from build123d import *

# Parameters (mm, degrees)
SKETCH1_W                = 40.386
SKETCH1_H                = 19.812
BOSS_EXTRUDE1_DEPTH      = 40.64
SKETCH2_W                = 19.812
SKETCH2_H                = 4
BOSS_EXTRUDE2_DEPTH      = 7
BOSS_EXTRUDE2_DEPTH_BACK = 47
SKETCH3_R                = 8.5
BOSS_EXTRUDE3_DEPTH      = 2
FILLET1_R                = 1
SKETCH4_R                = 2.117245373
BOSS_EXTRUDE4_DEPTH      = 5.2


with BuildPart() as part:
    # Sketch1 → Boss-Extrude1 (new body)
    with BuildSketch(Plane(origin=(0, 0, 0), x_dir=(1, 0, 0), z_dir=(0, 1, 0))):
        Rectangle(SKETCH1_W, SKETCH1_H)
    extrude(amount=BOSS_EXTRUDE1_DEPTH)

    # Sketch2 → Boss-Extrude2 (add, two sides)
    with BuildSketch(Plane(origin=(20.193, 0, 0), x_dir=(0, 0, -1), z_dir=(1, 0, 0))) as boss_extrude2_sk:
        with Locations((0, 25.94)):
            Rectangle(SKETCH2_W, SKETCH2_H)
    extrude(amount=BOSS_EXTRUDE2_DEPTH)
    extrude(boss_extrude2_sk.sketch, amount=-BOSS_EXTRUDE2_DEPTH_BACK)

    # Sketch3 → Boss-Extrude3 (add)
    with BuildSketch(Plane(origin=(0, 40.64, 0), x_dir=(1, 0, 0), z_dir=(0, 1, 0))):
        with Locations((10.018571985, 0)):
            Circle(SKETCH3_R)
    extrude(amount=BOSS_EXTRUDE3_DEPTH)

    # Fillet1
    fillet1_edges = [part.edges().sort_by_distance(p)[0] for p in [
        (1.518571985, 42.64, 0),
    ]]
    fillet(fillet1_edges, radius=FILLET1_R)

    # Sketch4 → Boss-Extrude4 (add)
    with BuildSketch(Plane(origin=(0, 42.64, 0), x_dir=(1, 0, 0), z_dir=(0, 1, 0))):
        with Locations((10.018571985, 0)):
            Circle(SKETCH4_R)
    extrude(amount=BOSS_EXTRUDE4_DEPTH)


solid = part.part
Can you work these out from the model? Positions are in its coordinate system, mm. A direction names the side the tool comes from. Coordinates: 2 decimals unless noted, no trailing zeros. Loops run counter-clockwise (first coordinate to the right, second up) from the corner with the lowest first, then second, coordinate; pieces in that order, holes last. Notation, with made-up numbers: M 82,0 L 140,0 A14 ccw 140,12 Z; hole C 10,-6 d8. An arc over 180 degrees is marked long. Answer as CSV lines item,"result". Start each with the question number.
1. Suppose I cut it at B-B, the plane x = 22.5. List the corners of the cut face in (y, z) for me.
2. For faces 1 (the face through (-23, 27.94, 0)), 2 (the face through (20.193, 34, 0)), 3 (the face through (-23, 23.94, 0)), 4 (the face through (12, 42.64, 2)), which set-ups out of +Z, -Z, +X, -X, +Y, -Y let a thin tool reach every point of the face, with its end or its side?
3. Suppose I cut it at C-C, the plane y = 38. List the corners of the cut face in (x, z) for me.
4. For pin 1 Ø7.5 at (x, z) = (24, -1) entering from -Y; pin 2 Ø3.5 at (x, z) = (-23.5, 0.5) entering from +Y; pin 3 Ø6 at (y, z) = (7, -5) entering from +X, each with a flat end and sliding along its axis, tell me the tip position at first contact or that it passes through.
5. If I drill on probe 1 along Y at (x, z) = (-8, 0); probe 2 along X at (y, z) = (12.5, 5); probe 3 along Y at (x, z) = (24, 4.5), over which ranges is the centre line in solid material (lowest first)? Write a range as [from, to].
6. Suppose I cut it at A-A, the plane z = 0. List the corners of the cut face in (x, y) for me, plus the area to 3 significant figures.
Output:
1,outline,"M 23.94,-9.91 L 27.94,-9.91 L 27.94,9.91 L 23.94,9.91 Z"
2,face 1,"+Z, -Z, -X, +Y"
2,face 2,"+Z, -Z, +X, +Y"
2,face 3,"+Z, -Z, -X, -Y"
2,face 4,"+Y"
3,outline,"M -20.19,-9.91 L 20.19,-9.91 L 20.19,9.91 L -20.19,9.91 Z"
4,pin 1,"stops at y = 23.94"
4,pin 2,"stops at y = 27.94"
4,pin 3,"stops at x = 20.19"
5,probe 1,"y = [0, 40.64]"
5,probe 2,"x = [-20.19, 20.19]"
5,probe 3,"y = [23.94, 27.94]"
6,outline,"M -26.81,23.94 L -20.19,23.94 L -20.19,0 L 20.19,0 L 20.19,23.94 L 27.19,23.94 L 27.19,27.94 L 20.19,27.94 L 20.19,40.64 L 18.52,40.64 L 18.52,41.64 A1 ccw 17.52,42.64 L 12.14,42.64 L 12.14,47.84 L 7.9,47.84 L 7.9,42.64 L 2.52,42.64 A1 ccw 1.52,41.64 L 1.52,40.64 L -20.19,40.64 L -20.19,27.94 L -26.81,27.94 Z"
6,area,"1,750 mm^2"
